Read the model definition and answer for the solid it produces. Units are mm, in the model's axes. A direction names the side the tool comes from. Give positions to 0.01 mm unless a question says otherwise; leave off trailing zeros. Order: outer loops, then holes, each group sorted by start corner. A loop starts at its lowest first (then second) coordinate and runs counter-clockwise, first axis right, second up. Notation, with made-up numbers: (24, 83.25) - (66, 83.25) arc R25 cw to (66, 99.25) - close; hole circle Ø1 at (-6, 48). An arc over 180 degrees is marked (long way). Write item = value, one per line.
```python
from build123d import *

# Parameters (mm, degrees)
SKETCH1_W           = 8.1026
SKETCH1_H           = 13.9954
BOSS_EXTRUDE1_DEPTH = 12.319
SKETCH2_R           = 3
SKETCH2_R_2         = 1.8034
BOSS_EXTRUDE2_DEPTH = 3.9878


with BuildPart() as part:
    # Sketch1 → Boss-Extrude1 (new body)
    with BuildSketch(Plane(origin=(0, 0, 0), x_dir=(1, 0, 0), z_dir=(0, 1, 0))):
        with Locations((0.8509, 6.9977)):
            Rectangle(SKETCH1_W, SKETCH1_H)
    extrude(amount=BOSS_EXTRUDE1_DEPTH)

    # Sketch2 → Boss-Extrude2 (add)
    with BuildSketch(Plane.XY):
        with Locations(Location((0, 7.0104, 0), (0, 0, 180))):
            Circle(SKETCH2_R)
        with Locations((0, 7.0104)):
            Circle(SKETCH2_R_2, mode=Mode.SUBTRACT)
    extrude(amount=BOSS_EXTRUDE2_DEPTH)


solid = part.part
```
1. Section C-C (x = -2) is taken. Determine the outline of the cut face in (y, z), and give its area (3 significant figures).
Recorded:
outline = (0, -14) - (12.32, -14) - (12.32, 0) - (9.25, 0) - (9.25, 3.99) - (4.77, 3.99) - (4.77, 0) - (0, 0) - close
area = 190 mm^2
2. For faces 4 (the face through (0, 7, 0)), 5 (the face through (1, 0, -7)), determine the directions among +Z, -Z, +X, -X, +Y, -Y from which every point of the face is accessible in a straight line to the end or side of a thin tool.
Recorded:
face_4 = +Z
face_5 = +Z, -Z, +X, -X, -Y
3. Section B-B (y = 4.25) is taken. Determine the outline of the cut face in (x, z).
Recorded:
outline = (-3.2, -14) - (4.9, -14) - (4.9, 0) - (1.17, 0) - (1.17, 3.99) - (-1.17, 3.99) - (-1.17, 0) - (-3.2, 0) - close
4. Section A-A (x = 0) is taken. Determine the outline of the cut face in (y, z).
Recorded:
outline = (0, -14) - (12.32, -14) - (12.32, 0) - (10.01, 0) - (10.01, 3.99) - (8.81, 3.99) - (8.81, 0) - (5.21, 0) - (5.21, 3.99) - (4.01, 3.99) - (4.01, 0) - (0, 0) - close
5. Section D-D (y = 5.5) is taken. Determine the outline of the cut face in (x, z), and give its area (3 significant figures).
Recorded:
outline = (-3.2, -14) - (4.9, -14) - (4.9, 0) - (2.59, 0) - (2.59, 3.99) - (0.99, 3.99) - (0.99, 0) - (-0.99, 0) - (-0.99, 3.99) - (-2.59, 3.99) - (-2.59, 0) - (-3.2, 0) - close
area = 126 mm^2
6. Straight lines are drawn through the part: L1, parallel to Y at x = 0, z = 2.2; L2, parallel to Z at x = -1.5, y = 4.25; L3, parallel to Y at x = 0.5, z = 2. For each, find the intervals that lie inside material, in ascending order. Write a range as [from, to].
Recorded:
L1 = [4.01, 5.21], [8.81, 10.01]
L2 = [-14, 0]
L3 = [4.05, 5.28], [8.74, 9.97]
7. Determine the mould class of faces 1 (the face through (1, 6, -13.995)), 2 (the face through (0.391, 4.036, 1.966)), 3 (the face through (0.97, 8.53, 1.97)) for opening direction X: +X half, -X half, draft (parallel to the pull), parting line (faces both ways), or undercut.
Recorded:
face_1 = draft
face_2 = parting line
face_3 = undercut
